The listing builds one solid part. Answer for the finished solid, in the listing's coordinates (mm). Face numbers are marked on the shaded views. A direction names the side the tool comes from. Round coordinates to 2 decimals unless told otherwise and drop trailing zeros. Write each loop counter-clockwise with the first axis right and the second up, starting at its lowest first coordinate (ties: lowest second). Pieces come first, ordered by that corner, then holes. Notation, with made-up numbers: (19.5, 36) - (51.5, 36) arc R19 ccw to (51.5, 56) - close; hole circle Ø6 at (71.25, 26). An arc over 180 degrees is marked (long way). Answer in a Markdown table with one row per item.
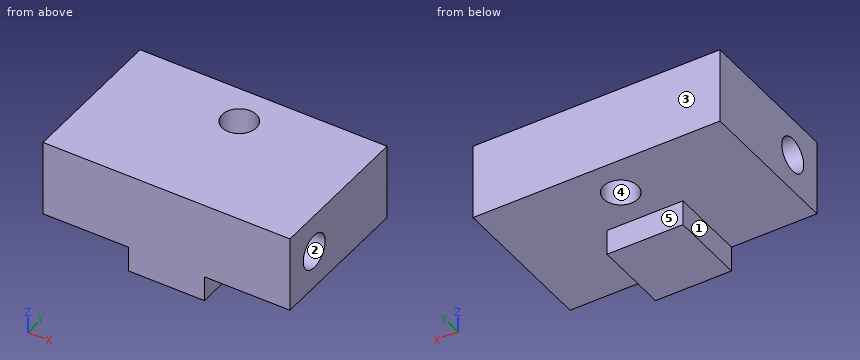
from build123d import *

# Parameters (mm, degrees)
F0_W     = 31
F0_H     = 19.05
F0_R     = 2.15265
F1_DEPTH = 9.525
F2_R     = 2.15265
F3_DEPTH = 31
F4_W     = 9.525
F4_H     = 9.525
F5_DEPTH = 3.175


with BuildPart() as f1:
    # F0 (on Top) → F1 (new body)
    with BuildSketch(Plane.XY):
        with Locations((15.5, -9.525)):
            Rectangle(F0_W, F0_H)
        with Locations((15.5, -4.7625)):
            Circle(F0_R, mode=Mode.SUBTRACT)
    extrude(amount=F1_DEPTH)

    # F2 (on face) → F3 (cut, through all)
    with BuildSketch(Plane.YZ.offset(31)):
        with Locations((-14.2875, 4.7625)):
            Circle(F2_R)
    extrude(amount=-F3_DEPTH, mode=Mode.SUBTRACT)

    # F4 (on face) → F5 (join)
    with BuildSketch(Plane(origin=(0, 0, 0), x_dir=(1, 0, 0), z_dir=(0, 0, -1))):
        with Locations((15.5, 14.2875)):
            Rectangle(F4_W, F4_H)
    extrude(amount=F5_DEPTH)


solid = f1.part
(1) Section A-A (x = 15.5) is taken. State how many separate pieces and enclosed holes the cut face has, and give its area (3 significant figures).
Checked values:
| item | result |
|---|---|
| separate pieces | 2 |
| enclosed holes | 1 |
| area | 156 mm2 |
(2) For the marked faces 4 and 5, determine the directions among +Z, -Z, +X, -X, +Y, -Y from which every point of the face is accessible in a straight line to the end or side of a thin tool.
Checked values:
| item | result |
|---|---|
| face 4 | +Z, -Z |
| face 5 | -Z, +X, -X, +Y |
(3) Find the intervals of material crossed by line 1 (Y direction, x = 15.5, z = 4.5); line 2 (Y direction, x = 15.5, z = 3.5); line 3 (Z direction, x = 24, y = -4.25) (3 decimals), in increasing order.
Checked values:
| item | result |
|---|---|
| line 1 | y = -19.05 to -16.42, -12.15 to -6.92, -2.61 to 0 |
| line 2 | y = -19.05 to -16.03, -12.54 to -6.92, -2.61 to 0 |
| line 3 | z = 0 to 9.525 |
(4) Section B-B (y = -13.25) is taken. Give the vertices of the cut face in (x, z) (1 decimal), and give its area (3 significant figures).
Checked values:
| item | result |
|---|---|
| outline | (0, 0) - (10.7, 0) - (10.7, -3.2) - (20.3, -3.2) - (20.3, 0) - (31, 0) - (31, 2.9) - (0, 2.9) - close; (0, 6.6) - (31, 6.6) - (31, 9.5) - (0, 9.5) - close |
| area | 209 mm2 |
(5) Section D-D (y = -4) is taken. Give the vertices of the cut face in (x, z) (3 decimals).
Checked values:
| item | result |
|---|---|
| outline | (0, 0) - (13.487, 0) - (13.487, 9.525) - (0, 9.525) - close; (17.513, 0) - (31, 0) - (31, 9.525) - (17.513, 9.525) - close |
(6) Flat-ended cylindrical pins translate along their axes: pin 1 (5.5 mm diameter, centred on x = 15.5, y = -4.76, fed in from -Z); pin 2 (2.5 mm diameter, centred on x = 14.5, z = -1.5, fed in from +Y) (3 decimals); pin 3 (1 mm diameter, centred on y = -15.5, z = -1, fed in from -X). Find the tip coordinate at first contact, or state that the pin passes through.
Checked values:
| item | result |
|---|---|
| pin 1 | stops at z = 0 |
| pin 2 | stops at y = -9.525 |
| pin 3 | stops at x = 10.74 |
(7) For a pull along Y with two mould halves and no side action, classify the marked faces 1, 2 and 3 as pulls with the +Y half, pulls with the -Y half, needs draft (parallel to the pull), parting line crosses it, or undercut.
Checked values:
| item | result |
|---|---|
| face 1 | needs draft |
| face 2 | undercut |
| face 3 | pulls with the +Y half |
